```python
from build123d import *

# Parameters (mm, degrees)
BOSS_EXTRUDE1_DEPTH      = 2.5
SKETCH2_R                = 9.5
BOSS_EXTRUDE2_DEPTH      = 3
SKETCH3_R                = 16
BOSS_EXTRUDE3_DEPTH      = 5
BOSS_EXTRUDE3_DEPTH_BACK = 0.25


with BuildPart() as part:
    # Sketch1 → Boss-Extrude1 (new body)
    with BuildSketch(Plane.XY):
        with BuildLine():
            Line((5.417779502, 13.449820269), (3.549579674, 8.811951211))
            ThreePointArc((3.549579674, 8.811951211), (-1.94104371, 9.299588664), (-6.778170146, 6.656305993))
            Line((-6.778170146, 6.656305993), (-10.345628118, 10.159624937))
            ThreePointArc((-10.345628118, 10.159624937), (-12.131657575, 7.941843897), (-13.449820269, 5.417779502))
            Line((-13.449820269, 5.417779502), (-8.811951211, 3.549579674))
            ThreePointArc((-8.811951211, 3.549579674), (-9.299588664, -1.94104371), (-6.656305993, -6.778170146))
            Line((-6.656305993, -6.778170146), (-10.159624937, -10.345628118))
            ThreePointArc((-10.159624937, -10.345628118), (-7.941843897, -12.131657575), (-5.417779502, -13.449820269))
            Line((-5.417779502, -13.449820269), (-3.549579674, -8.811951211))
            ThreePointArc((-3.549579674, -8.811951211), (1.94104371, -9.299588664), (6.778170146, -6.656305993))
            Line((6.778170146, -6.656305993), (10.345628118, -10.159624937))
            ThreePointArc((10.345628118, -10.159624937), (12.131657575, -7.941843897), (13.449820269, -5.417779502))
            Line((13.449820269, -5.417779502), (8.811951211, -3.549579674))
            ThreePointArc((8.811951211, -3.549579674), (9.299588664, 1.94104371), (6.656305993, 6.778170146))
            Line((6.656305993, 6.778170146), (10.159624937, 10.345628118))
            ThreePointArc((10.159624937, 10.345628118), (7.941843897, 12.131657575), (5.417779502, 13.449820269))
        make_face()
    extrude(amount=BOSS_EXTRUDE1_DEPTH)

    # Sketch2 → Boss-Extrude2 (add)
    with BuildSketch(Plane.XY.offset(2.5)):
        Circle(SKETCH2_R)
    extrude(amount=BOSS_EXTRUDE2_DEPTH)

    # Sketch3 → Boss-Extrude3 (add, two sides)
    with BuildSketch(Plane.XY.offset(5.5)) as boss_extrude3_sk:
        Circle(SKETCH3_R)
    extrude(amount=BOSS_EXTRUDE3_DEPTH)
    extrude(boss_extrude3_sk.sketch, amount=-BOSS_EXTRUDE3_DEPTH_BACK)


solid = part.part
```
Model file for the job. Use its own axes, mm. A direction names the side the tool comes from. Give positions to 0.01 mm unless a question says otherwise; leave off trailing zeros. Loops run counter-clockwise (first coordinate to the right, second up) from the corner with the lowest first, then second, coordinate; pieces in that order, holes last. Notation, with made-up numbers: (3.25, 29) - (55.25, 29) arc R27 ccw to (55.25, 58) - close; hole circle Ø2 at (-24, -36.75). An arc over 180 degrees is marked (long way). One line per item, written item: value. Start each with the question number.
1. Slice it at B-B (z = 1.25). List the corners of the cut face in (x, y).
2. Probe L1, parallel to Z at x = -11.5, y = 5.5; L2, parallel to Z at x = 2, y = 11; L3, parallel to Y at x = -7, z = 2.25. List the from-to ranges inside material, lowest first. Write a range as from..to.
3. Pin check, flat tips, straight feed: pin 1 (2 mm diameter, centred on x = -7, y = -2, fed in from -Z); pin 2 (3 mm diameter, centred on y = 9, z = 7.5, fed in from +X); pin 3 (4 mm diameter, centred on y = 11.5, z = 6.5, fed in from -X); pin 4 (2 mm diameter, centred on x = -5.5, z = 6, fed in from +Y). Stop position of each tip, or through.
4. Slice it at A-A (x = 0). List the corners of the cut face in (y, z).
5. Which spindle directions (+Z, -Z, +X, -X, +Y, -Y) get a long thin tool onto all of the face, cutting with end or side? Do faces 1 (the cylindrical face through (-12.11, 7.975, 1.232)), 2 (the flat face through (10, -7, 2.5)), 3 (the flat face through (-7, -10, 2.5)). Say none if no direction does.
6. Pull direction X, two halves, no side cores. Call faces 4 (the flat face through (-8.537, 8.383, 1.232)), 5 (the flat face through (7, 10, 2.5)), 6 (the flat face through (-8.383, -8.537, 1.232)): pulls with the +X half, pulls with the -X half, needs draft (parallel to the pull), parting line crosses it, or undercut.
7. Slice it at C-C (y = -7.5). List the corners of the cut face in (x, z).
Solution:
1. outline: (-13.45, 5.42) - (-8.81, 3.55) arc R9.5 ccw to (-6.66, -6.78) - (-10.16, -10.35) arc R14.5 ccw to (-5.42, -13.45) - (-3.55, -8.81) arc R9.5 ccw to (6.78, -6.66) - (10.35, -10.16) arc R14.5 ccw to (13.45, -5.42) - (8.81, -3.55) arc R9.5 ccw to (6.66, 6.78) - (10.16, 10.35) arc R14.5 ccw to (5.42, 13.45) - (3.55, 8.81) arc R9.5 ccw to (-6.78, 6.66) - (-10.35, 10.16) arc R14.5 ccw to start
2. L1: z = 0..2.5, 5.25..10.5
2. L2: z = 5.25..10.5
2. L3: y = -12.7..-7.13, -6.42..6.87
3. pin 1: stops at z = 0
3. pin 2: stops at x = 14.13
3. pin 3: stops at x = -12.87
3. pin 4: stops at y = 15.35
4. outline: (-16, 5.25) - (-9.5, 5.25) - (-9.5, 0) - (9.5, 0) - (9.5, 5.25) - (16, 5.25) - (16, 10.5) - (-16, 10.5) - close
5. face 1: -Z, -X, +Y
5. face 2: +X, -Y
5. face 3: -X, -Y
6. face 4: undercut
6. face 5: needs draft
6. face 6: pulls with the -X half
7. outline: (-14.13, 5.25) - (-5.83, 5.25) - (-5.83, 2.5) - (-7.37, 2.5) - (-7.37, 0) - (5.83, 0) - (5.83, 5.25) - (14.13, 5.25) - (14.13, 10.5) - (-14.13, 10.5) - close; (7.64, 0) - (12.41, 0) - (12.41, 2.5) - (7.64, 2.5) - close
